Could you check a few things on this drawing? It's one solid part, dimensions in mm from its lowest x, y, z. Coordinates: 2 decimals unless noted, no trailing zeros. Write each loop counter-clockwise with the first axis right and the second up, starting at its lowest first coordinate (ties: lowest second). Pieces come first, ordered by that corner, then holes. Notation, with made-up numbers: (15.25, 14.25) - (41.25, 14.25) arc R24 ccw to (41.25, 34.25) - close; hole circle Ø8 at (27.25, 70). An arc over 180 degrees is marked (long way). Use one line per item in the form item = value. Start each with the question number.
(1) If we section it at D-D on z = 37: Please give me the cut outline in (x, y).
(2) If we section it at C-C on y = 1.15: Please give me the cut outline in (x, z), then the cut area to 3 significant figures.
(3) If I drill on probe 1 along Z at (x, y) = (50.5, 0.6); probe 2 along X at (y, z) = (0.7, 50.5), over which ranges is the centre line in solid material (lowest first)? Write a range as from..to.
(4) If we section it at A-A on x = 20: Please give me the cut outline in (y, z), then the cut area to 3 significant figures.
(5) If we section it at B-B on z = 50.5: Please give me the cut outline in (x, y), then the cut area to 3 significant figures.
(6) For pin 1 Ø0.7 at (x, y) = (47, 1) entering from +Z, with a flat end and sliding along its axis, tell me the tip position at first contact or that it passes through.
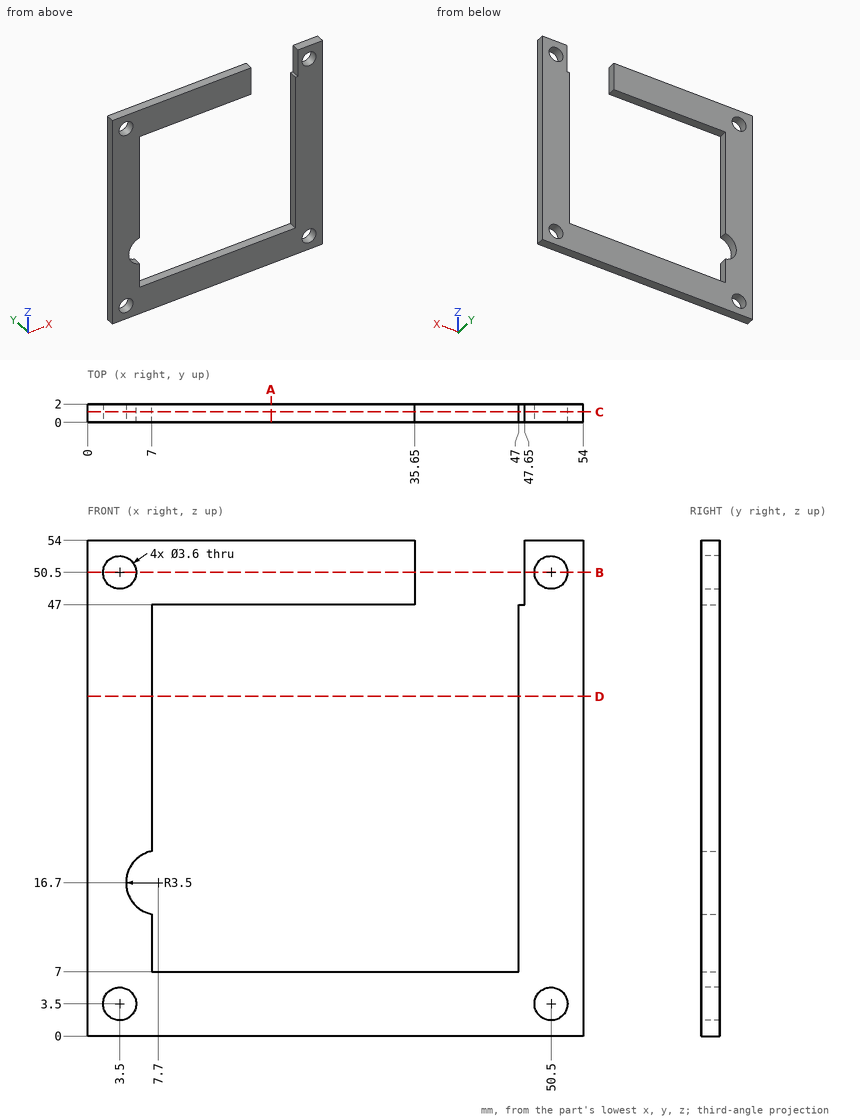
Reported:
q1.outline = (0, 0) - (7, 0) - (7, 2) - (0, 2) - close; (47, 0) - (54, 0) - (54, 2) - (47, 2) - close
q2.outline = (0, 0) - (54, 0) - (54, 54) - (47.65, 54) - (47.65, 47) - (47, 47) - (47, 7) - (7, 7) - (7, 13.27) arc R3.5 cw to (7, 20.13) - (7, 47) - (35.65, 47) - (35.65, 54) - (0, 54) - close; hole circle Ø3.6 at (3.5, 3.5); hole circle Ø3.6 at (3.5, 50.5); hole circle Ø3.6 at (50.5, 3.5); hole circle Ø3.6 at (50.5, 50.5)
q2.area = 1,180 mm2
q3.probe_1 = 0..1.7, 5.3..48.7, 52.3..54
q3.probe_2 = 0..1.7, 5.3..35.65, 47.65..48.7, 52.3..54
q4.outline = (0, 0) - (2, 0) - (2, 7) - (0, 7) - close; (0, 47) - (2, 47) - (2, 54) - (0, 54) - close
q4.area = 28.0 mm2
q5.outline = (0, 0) - (1.7, 0) - (1.7, 2) - (0, 2) - close; (5.3, 0) - (35.65, 0) - (35.65, 2) - (5.3, 2) - close; (47.65, 0) - (48.7, 0) - (48.7, 2) - (47.65, 2) - close; (52.3, 0) - (54, 0) - (54, 2) - (52.3, 2) - close
q5.area = 69.6 mm2
q6.pin_1 = 47
